Verification items for the finished model (mm, model axes). A direction names the side the tool comes from. Coordinates: 2 decimals unless noted, no trailing zeros. Order: outer loops, then holes, each group sorted by start corner. A loop starts at its lowest first (then second) coordinate and runs counter-clockwise, first axis right, second up. Notation, with made-up numbers: (84.25, 73) -> (110.25, 73) arc R15 ccw to (110.25, 81) -> close; hole circle Ø5 at (61.5, 83). An arc over 180 degrees is marked (long way). Write item = value, one per line. Start each with the question number.
1. Cross-section at D-D on y = 20. Record the cut outline in (x, z), plus the area to 3 significant figures.
2. Cross-section at A-A on z = 171.45. Record the cut outline in (x, y), plus the area to 3 significant figures.
3. Cross-section at C-C on x = 2.5. Record the cut outline in (y, z).
4. Go/stop test with flat-tipped pins: P1, Ø13.5, axis at x = 6.5, y = -23.5, coming from the +Z side; P2, Ø1.5, axis at x = -65.5, y = 96, coming from the -Z side; P3, Ø6, axis at x = 80.07, z = 171.45, coming from the +Y side. Record where each tip stops, or that it passes through.
5. Release check for a two-part mould opening along X. For faces 6 (the flat face through (-91.382, 75, 2)), 7 (the flat face through (105.468, -11, 3)), 8 (the flat face through (5, 126, 190.5)) record: +X half, -X half, draft (parallel to the pull), parting line (faces both ways), or undercut.
6. Cross-section at B-B on z = 0. Record the cut outline in (x, y).
7. Thickness scan on line 1 along X through (y, z) = (125, -171); line 2 along Z through (x, y) = (83, 124); line 3 along Y through (x, z) = (21, -170.5). Record the ranges inside material, lowest first. Write a range as from..to.
8. Set-up check for faces 1 (the cylindrical face through (-72.1, 125.72, -176.65)), 2 (the flat face through (5, -19, -177.8)), 3 (the cylindrical face through (102.337, 7.056, 2.723)), 4 (the flat face through (5, 3.852, 130)), 5 (the flat face through (5, 3.852, -132)): record each of +Z, -Z, +X, -X, +Y, -Y from which the full face is reachable in a straight line by a thin tool's end or side.
from build123d import *

# Parameters (mm, degrees)
BOSS_EXTRUDE1_DEPTH  = 4
SKETCH2_R            = 5.75
CUT_EXTRUDE1_DEPTH   = 3.75
SKETCH5_R            = 0.205
CUT_EXTRUDE2_DEPTH   = 0.41
LPATTERN1_COUNT      = 4
LPATTERN1_PITCH      = 2
LPATTERN1_COUNT_DIR2 = 2
LPATTERN1_PITCH_DIR2 = 13.5
CUT_EXTRUDE3_DEPTH   = 13.440483311
CUT_EXTRUDE4_REACH   = 14.44
SKETCH6_3_R          = 4.875
SKETCH6_3_R_2        = 0.75
SCALE1_SCALE         = 25.4


with BuildPart() as part:
    # Sketch1 → Boss-Extrude1 (new, symmetric)
    with BuildSketch(Plane(origin=(0, 0, 0), x_dir=(0, 0, -1), z_dir=(1, 0, 0))):
        with BuildLine():
            Line((-7, 0.875), (-7, -0.875))
            Line((-7, -0.875), (7, -0.875))
            Line((7, -0.875), (7, 0.875))
            Line((7, 0.875), (3.31662479, 0.875))
            ThreePointArc((3.31662479, 0.875), (5.186676874, 2.858647401), (5.985975276, 5.465))
            Line((5.985975276, 5.465), (7.5, 5.465))
            Line((7.5, 5.465), (7.5, 5.875))
            Line((7.5, 5.875), (-7.5, 5.875))
            Line((-7.5, 5.875), (-7.5, 5.465))
            Line((-7.5, 5.465), (-5.985975276, 5.465))
            ThreePointArc((-5.985975276, 5.465), (-5.186676874, 2.858647401), (-3.31662479, 0.875))
            Line((-3.31662479, 0.875), (-7, 0.875))
        make_face()
    extrude(amount=BOSS_EXTRUDE1_DEPTH, both=True)

    # Sketch2 → Cut-Extrude1 (cut, symmetric)
    with BuildSketch(Plane(origin=(0, 0, 0), x_dir=(0, 0, -1), z_dir=(1, 0, 0))):
        with Locations((0, 5.875)):
            Circle(SKETCH2_R)
    extrude(amount=CUT_EXTRUDE1_DEPTH, both=True, mode=Mode.SUBTRACT)

    # Sketch5 → Cut-Extrude2 (cut)
    with BuildSketch(Plane(origin=(0, 5.875, 0), x_dir=(1, 0, 0), z_dir=(0, 1, 0))):
        with Locations(Location((-3, 6.75, 0), (0, 0, 270))):
            Circle(SKETCH5_R)
    cut_extrude2 = extrude(amount=-CUT_EXTRUDE2_DEPTH, mode=Mode.SUBTRACT)

    # LPattern1: Cut-Extrude2 4 × 2
    with Locations(*[(i * LPATTERN1_PITCH, 0, j * LPATTERN1_PITCH_DIR2) for i in range(LPATTERN1_COUNT) for j in range(LPATTERN1_COUNT_DIR2) if (i, j) != (0, 0)]):
        add(cut_extrude2, mode=Mode.SUBTRACT)

    # Sketch6 → Cut-Extrude3 (cut, through all)
    with BuildSketch(Plane(origin=(4, 0, 0), x_dir=(0, 0, -1), z_dir=(1, 0, 0))):
        with BuildLine():
            Line((-0.75, 5.875), (0.75, 5.875))
            ThreePointArc((0.75, 5.875), (0, 6.625), (-0.75, 5.875))
        make_face()
        with BuildLine():
            ThreePointArc((-0.75, 5.875), (0, 5.125), (0.75, 5.875))
            Line((0.75, 5.875), (-0.75, 5.875))
        make_face()
    extrude(amount=-CUT_EXTRUDE3_DEPTH, mode=Mode.SUBTRACT)

    # Sketch6<3> → Cut-Extrude4 (cut, up to next)
    with BuildSketch(Plane(origin=(4, 0, 0), x_dir=(0, 0, -1), z_dir=(1, 0, 0)), mode=Mode.PRIVATE) as cut_extrude4_sk1:
        with Locations((0, 5.875)):
            Circle(SKETCH6_3_R)
        with Locations((0, 5.875)):
            Circle(SKETCH6_3_R_2, mode=Mode.SUBTRACT)
    cut_extrude4_tool1 = extrude(cut_extrude4_sk1.sketch, amount=-CUT_EXTRUDE4_REACH, mode=Mode.PRIVATE) & part.part
    add(cut_extrude4_tool1.solids().sort_by_distance((4, 5.875, 4.737114))[0], mode=Mode.SUBTRACT)


with BuildPart() as part_1:
    # Scale1: scaled about (-0.158509588, 0.753010739, 0)
    add(part.part.scale(SCALE1_SCALE).moved(Location((3.867633947, -18.373462032, 0))))


solid = part_1.part
Worked out:
q1.outline = (-97.73, -104.58) -> (105.47, -104.58) -> (105.47, -55.18) -> (99.12, -55.18) -> (99.12, -95.09) -> (-91.38, -95.09) -> (-91.38, 95.09) -> (99.12, 95.09) -> (99.12, 55.18) -> (105.47, 55.18) -> (105.47, 104.58) -> (-97.73, 104.58) -> close
q1.area = 5,570 mm²
q2.outline = (-97.73, -40.6) -> (105.47, -40.6) -> (105.47, 3.85) -> (-97.73, 3.85) -> close; (-97.73, 120.44) -> (-77.54, 120.44) -> (-77.54, 130.85) -> (-97.73, 130.85) -> close; (-67.13, 120.44) -> (-26.74, 120.44) -> (-26.74, 130.85) -> (-67.13, 130.85) -> close; (-16.33, 120.44) -> (24.06, 120.44) -> (24.06, 130.85) -> (-16.33, 130.85) -> close; (34.47, 120.44) -> (74.86, 120.44) -> (74.86, 130.85) -> (34.47, 130.85) -> close; (85.27, 120.44) -> (105.47, 120.44) -> (105.47, 130.85) -> (85.27, 130.85) -> close
q2.area = 10,700 mm²
q3.outline = (-40.6, -177.8) -> (3.85, -177.8) -> (3.85, -84.24) arc R152.4 ccw to (120.44, -152.04) -> (120.44, -190.5) -> (130.85, -190.5) -> (130.85, -146.05) arc R146.05 cw to (130.85, 146.05) -> (130.85, 190.5) -> (120.44, 190.5) -> (120.44, 152.04) arc R152.4 ccw to (3.85, 84.24) -> (3.85, 177.8) -> (-40.6, 177.8) -> close
q4.P1 = 177.8
q4.P2 = -148.54
q4.P3 = 3.85
q5.face_6 = undercut
q5.face_7 = +X half
q5.face_8 = draft
q6.outline = (-97.73, -40.6) -> (105.47, -40.6) -> (105.47, 7.03) -> (99.12, 7.03) -> (99.12, -15.2) -> (-91.38, -15.2) -> (-91.38, 111.8) -> (-97.73, 111.8) -> close
q7.line_1 = -97.73..-77.52, -67.14..-26.72, -16.34..24.08, 34.46..74.88, 85.26..105.47
q7.line_2 = -190.5..-175.75, -167.15..-145.89, 145.89..167.15, 175.75..190.5
q7.line_3 = -40.6..3.85, 120.44..130.85
q8.face_1 = +Y
q8.face_2 = -Z, +X, -X, -Y
q8.face_3 = +X, +Y
q8.face_4 = +Z, +X, -X
q8.face_5 = -Z, +X, -X
